from build123d import *

# Parameters (mm, degrees)
ESQUISSE1_W              = 200
ESQUISSE1_H              = 140
BOSS_EXTRU_1_DEPTH       = 6
ESQUISSE2_R              = 9
ESQUISSE2_R_2            = 4
ESQUISSE2_W              = 6.5
ESQUISSE2_H              = 20
ESQUISSE2_W_2            = 12.5
ESQUISSE2_H_2            = 28.5
ENL_V_MAT_EXTRU_1_DEPTH  = 245.204832057
ESQUISSE3_W              = 40
ESQUISSE3_H              = 6
ESQUISSE3_W_2            = 66.5
ENL_V_MAT_EXTRU_2_DEPTH  = 6
ESQUISSE7_W              = 6
ESQUISSE7_H              = 128
ESQUISSE7_H_2            = 14
ESQUISSE7_R              = 1.5
ENL_V_MAT_EXTRU_4_DEPTH  = 6
ESQUISSE9_W              = 5.785245128
ESQUISSE9_H              = 20
ENL_V_MAT_EXTRU_5_DEPTH  = 6
ESQUISSE12_W             = 6
ESQUISSE12_H             = 40
BOSS_EXTRU_2_DEPTH       = 6
ESQUISSE13_R             = 1.5
ENL_V_MAT_EXTRU_7_DEPTH  = 6
ESQUISSE14_R             = 1.5
ESQUISSE14_W             = 15
ESQUISSE14_H             = 6
ENL_V_MAT_EXTRU_8_DEPTH  = 245.204832057
ESQUISSE15_R             = 1.5
ENL_V_MAT_EXTRU_9_DEPTH  = 245.204832057
ESQUISSE17_R             = 3
ENL_V_MAT_EXTRU_12_DEPTH = 3
ESQUISSE18_R             = 1.5
ESQUISSE18_W             = 15
ESQUISSE18_H             = 6
ENL_V_MAT_EXTRU_13_DEPTH = 245.204832057
ESQUISSE16_R             = 2.995
ESQUISSE16_R_2           = 3
ENL_V_MAT_EXTRU_11_DEPTH = 3


with BuildPart() as part:
    # Esquisse1 → Boss.-Extru.1 (new body)
    with BuildSketch(Plane.XY):
        with Locations((-100, 70)):
            Rectangle(ESQUISSE1_W, ESQUISSE1_H)
    extrude(amount=BOSS_EXTRU_1_DEPTH)

    # Esquisse2 → Enlèv. mat.-Extru.1 (cut, through all)
    with BuildSketch(Plane.XY.offset(6)):
        with Locations((-20, 92)):
            Circle(ESQUISSE2_R)
        with Locations((-180, 87)):
            Circle(ESQUISSE2_R_2)
        with Locations((-180, 42.75)):
            Rectangle(ESQUISSE2_W, ESQUISSE2_H)
        with Locations((-20, 42.75)):
            Rectangle(ESQUISSE2_W_2, ESQUISSE2_H_2)
    extrude(amount=-ENL_V_MAT_EXTRU_1_DEPTH, mode=Mode.SUBTRACT)

    # Esquisse3 → Enlèv. mat.-Extru.2 (cut)
    with BuildSketch(Plane.XY.offset(6)):
        with Locations((-180, 3)):
            Rectangle(ESQUISSE3_W, ESQUISSE3_H)
        with Locations((-100, 3)):
            Rectangle(ESQUISSE3_W, ESQUISSE3_H)
        with Locations((-20, 3)):
            Rectangle(ESQUISSE3_W, ESQUISSE3_H)
        with Locations((-166.75, 137)):
            Rectangle(ESQUISSE3_W_2, ESQUISSE3_H)
        with Locations((-33.25, 137)):
            Rectangle(ESQUISSE3_W_2, ESQUISSE3_H)
    extrude(amount=-ENL_V_MAT_EXTRU_2_DEPTH, mode=Mode.SUBTRACT)

    # Esquisse7 → Enlèv. mat.-Extru.4 (cut)
    with BuildSketch(Plane.XY.offset(6)):
        with Locations((-197, 70)):
            Rectangle(ESQUISSE7_W, ESQUISSE7_H)
        with Locations((-3, 127)):
            Rectangle(ESQUISSE7_W, ESQUISSE7_H_2)
        with Locations((-3, 13)):
            Rectangle(ESQUISSE7_W, ESQUISSE7_H_2)
        with Locations((-3, 40)):
            Circle(ESQUISSE7_R)
        with Locations((-3, 100)):
            Circle(ESQUISSE7_R)
    extrude(amount=-ENL_V_MAT_EXTRU_4_DEPTH, mode=Mode.SUBTRACT)

    # Esquisse9 → Enlèv. mat.-Extru.5 (cut)
    with BuildSketch(Plane.XY.offset(6)):
        with Locations((-2.892622564, 70)):
            Rectangle(ESQUISSE9_W, ESQUISSE9_H)
    extrude(amount=-ENL_V_MAT_EXTRU_5_DEPTH, mode=Mode.SUBTRACT)

    # Esquisse12 → Boss.-Extru.2 (add)
    with BuildSketch(Plane.XY.offset(6)):
        with Locations((-197, 100)):
            Rectangle(ESQUISSE12_W, ESQUISSE12_H)
        with Locations((-197, 40)):
            Rectangle(ESQUISSE12_W, ESQUISSE12_H)
    extrude(amount=-BOSS_EXTRU_2_DEPTH)

    # Esquisse13 → Enlèv. mat.-Extru.7 (cut)
    with BuildSketch(Plane.XY.offset(6)):
        with Locations((-197, 100)):
            Circle(ESQUISSE13_R)
        with Locations((-197, 40)):
            Circle(ESQUISSE13_R)
    extrude(amount=-ENL_V_MAT_EXTRU_7_DEPTH, mode=Mode.SUBTRACT)

    # Esquisse14 → Enlèv. mat.-Extru.8 (cut, through all)
    with BuildSketch(Plane.XY.offset(6)):
        with Locations((-152.5, 72)):
            Circle(ESQUISSE14_R)
        with Locations((-142.5, 72)):
            Circle(ESQUISSE14_R)
        with Locations((-57.5, 72)):
            Circle(ESQUISSE14_R)
        with Locations((-47.5, 72)):
            Circle(ESQUISSE14_R)
        with Locations((-70, 72)):
            Rectangle(ESQUISSE14_W, ESQUISSE14_H)
        with Locations((-130, 72)):
            Rectangle(ESQUISSE14_W, ESQUISSE14_H)
    extrude(amount=-ENL_V_MAT_EXTRU_8_DEPTH, mode=Mode.SUBTRACT)

    # Esquisse15 → Enlèv. mat.-Extru.9 (cut, through all)
    with BuildSketch(Plane.XY.offset(6)):
        with Locations((-180, 93.5)):
            Circle(ESQUISSE15_R)
        with Locations((-180, 78.5)):
            Circle(ESQUISSE15_R)
    extrude(amount=-ENL_V_MAT_EXTRU_9_DEPTH, mode=Mode.SUBTRACT)

    # Esquisse17 → Enlèv. mat.-Extru.12 (cut)
    with BuildSketch(Plane.XY.offset(6)):
        with Locations((-180, 93.5)):
            Circle(ESQUISSE17_R)
        with Locations((-180, 78.5)):
            Circle(ESQUISSE17_R)
    extrude(amount=-ENL_V_MAT_EXTRU_12_DEPTH, mode=Mode.SUBTRACT)

    # Esquisse18 → Enlèv. mat.-Extru.13 (cut, through all)
    with BuildSketch(Plane.XY.offset(6)):
        with Locations((-117.5, 107)):
            Circle(ESQUISSE18_R)
        with Locations((-82.5, 107)):
            Circle(ESQUISSE18_R)
        with Locations((-117.5, 33)):
            Circle(ESQUISSE18_R)
        with Locations((-82.5, 33)):
            Circle(ESQUISSE18_R)
        with Locations((-127.5, 107)):
            Circle(ESQUISSE18_R)
        with Locations((-72.5, 107)):
            Circle(ESQUISSE18_R)
        with Locations((-72.5, 33)):
            Circle(ESQUISSE18_R)
        with Locations((-127.5, 33)):
            Circle(ESQUISSE18_R)
        with Locations((-100, 107)):
            Rectangle(ESQUISSE18_W, ESQUISSE18_H)
        with Locations((-100, 33)):
            Rectangle(ESQUISSE18_W, ESQUISSE18_H)
    extrude(amount=-ENL_V_MAT_EXTRU_13_DEPTH, mode=Mode.SUBTRACT)

    # Esquisse16 → Enlèv. mat.-Extru.11 (cut)
    with BuildSketch(Plane.XY.offset(6)):
        with Locations((-197, 100)):
            Circle(ESQUISSE16_R)
        with Locations((-142.5, 72)):
            Circle(ESQUISSE16_R_2)
        with Locations((-152.5, 72)):
            Circle(ESQUISSE16_R_2)
        with Locations((-57.5, 72)):
            Circle(ESQUISSE16_R_2)
        with Locations((-197, 40)):
            Circle(ESQUISSE16_R)
        with Locations(Location((-3, 40, 0), (0, 0, 180))):
            Circle(ESQUISSE16_R)
        with Locations(Location((-47.5, 72, 0), (0, 0, 180))):
            Circle(ESQUISSE16_R_2)
        with Locations(Location((-3, 100, 0), (0, 0, 180))):
            Circle(ESQUISSE16_R)
    extrude(amount=-ENL_V_MAT_EXTRU_11_DEPTH, mode=Mode.SUBTRACT)


solid = part.part
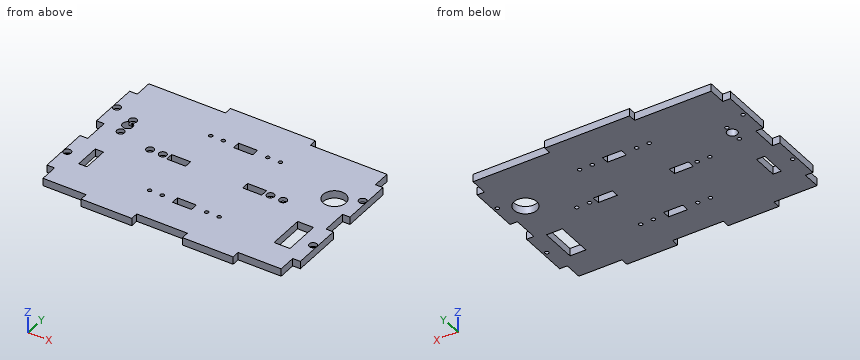
Can you work these out from the model? Positions are in its coordinate system, mm. Give positions to 0.01 mm unless a question says otherwise; leave off trailing zeros. Order: outer loops, then holes, each group sorted by start corner. A loop starts at its lowest first (then second) coordinate and runs counter-clockwise, first axis right, second up. Notation, with made-up numbers: (89, 3.5) - (144, 3.5) arc R14 ccw to (144, 16.5) - close; hole circle Ø5 at (77, 22). An arc over 180 degrees is marked (long way). Write each question's results on one line, items separated by ' | '.
1) Please list where these lines run through material, in increasing order: line 1 along Y through (x, z) = (-3, 5.35) (3 decimals); line 2 along Y through (x, z) = (-82.5, 2.85); line 3 along Y through (x, z) = (-105, 1.35). Write a range as [from, to].
Final values:
line 1: y = [20, 37.005], [42.995, 60], [80, 97.005], [102.995, 120] | line 2: y = [6, 31.5], [34.5, 105.5], [108.5, 140] | line 3: y = [6, 30], [36, 104], [110, 140]
2) Suppose I cut it at C-C, the plane y = 16. Write out the boundary of the cut face in (x, z).
Final values:
outline: (-194, 0) - (-6, 0) - (-6, 6) - (-194, 6) - close
3) I'm going to push flat-ended pins straight in: pin 1 Ø3.5 at (x, y) = (-47.5, 72) entering from +Z; pin 2 Ø2.5 at (x, y) = (-127.5, 107) entering from +Z; pin 3 Ø2 at (y, z) = (27.5, 4.5) entering from +X; pin 4 Ø3 at (x, z) = (-103, 3) entering from -Y. Where does each tip first touch, or does it pass through?
Final values:
pin 1: stops at z = 3 | pin 2: passes through | pin 3: stops at x = 0 | pin 4: stops at y = 6
4) Suppose I cut it at B-B, the plane x = -20. Write out the boundary of the cut face in (y, z), then the cut area to 3 significant figures.
Final values:
outline: (6, 0) - (28.5, 0) - (28.5, 6) - (6, 6) - close; (57, 0) - (83, 0) - (83, 6) - (57, 6) - close; (101, 0) - (134, 0) - (134, 6) - (101, 6) - close | area: 489 mm^2
5) Suppose I cut it at D-D, the plane z = 4.9. Give the number of separate pieces and of enclosed holes in the cut face, then the cut area to 3 significant figures.
Final values:
separate pieces: 1 | enclosed holes: 25 | area: 24,400 mm^2
6) Suppose I cut it at A-A, the plane x = -101.5. Write out the boundary of the cut face in (y, z), then the cut area to 3 significant figures.
Final values:
outline: (6, 0) - (30, 0) - (30, 6) - (6, 6) - close; (36, 0) - (104, 0) - (104, 6) - (36, 6) - close; (110, 0) - (140, 0) - (140, 6) - (110, 6) - close | area: 732 mm^2
